Design review of the part built by this model. Coordinates are the model's own, in mm. A direction names the side the tool comes from. Coordinates: 2 decimals unless noted, no trailing zeros. Write each loop counter-clockwise with the first axis right and the second up, starting at its lowest first coordinate (ties: lowest second). Pieces come first, ordered by that corner, then holes. Notation, with made-up numbers: (-37.75, 23) - (4.25, 23) arc R22 cw to (4.25, 57) - close; hole circle Ø6 at (45, 54.25). An arc over 180 degrees is marked (long way). Answer as CSV lines item,"result". Start each with the question number.
Q1. Mouldability with a two-part tool opening along Y and no side actions: class faces 4 (the face through (25, -15, 5)), 5 (the face through (-15, -25, 5)), 6 (the face through (-19, -8, 5)) as pulls with the +Y half, pulls with the -Y half, needs draft (parallel to the pull), parting line crosses it, or undercut.
Q2. For line 1 along X through (y, z) = (-18.5, 5); line 2 along Y through (x, z) = (8, 7.25), list the stretches that pass through material, from the lowest coordinate up. Write a range as [from, to].
Q3. Machinability: for faces 1 (the face through (-5.1, -22, 5)), 2 (the face through (15, -25, 5)), 3 (the face through (-10.5, -17, 5)), which of the approach directions +Z, -Z, +X, -X, +Y, -Y give a long, thin tool a straight path to every point of the face, cutting with its end or side? Answer none if there is none.
Q4. We need section A-A (y = 20.5). Write out the cut boundary in (x, z), plus the area to 3 significant figures.
Q5. Clearance check with a flat-ended pin moving along its axis: pin 1 (6 mm diameter, centred on x = 0, z = 2.5, fed in from +Y). State where the tip first meets the part, or that it passes through.
Q6. We need section B-B (x = -18). Write out the cut boundary in (y, z).
Autodesk Inventor part; units mm, degrees
ref_plane "YZ Plane" through (0, 0, 0) normal (1, 0, 0) x (0, 1, 0)
ref_plane "XZ Plane" through (0, 0, 0) normal (0, 1, 0) x (-1, 0, 0)
ref_plane "XY Plane" through (0, 0, 0) normal (0, 0, 1) x (1, 0, 0)
sketch "Sketch2" plane through (0, 0, 0) normal (0, 0, 1) x (1, 0, 0)
  line L0 (0, 0) -> (0, 6) construction
  circle A0 centre (0, 0) radius 6 construction
  circle A1 centre (0, 0) radius 7 construction
  arc A2 (1.1705, 5.8847) -> (-1.1705, 5.8847) centre (0, 0) ccw
  line L1 (-1.3656, 6.8655) -> (0, 0) construction
  line L2 (-1.3656, 6.8655) -> (-1.1705, 5.8847)
  arc A3 (-1.3656, 6.8655) -> (-3.889, 5.8203) centre (0, 0) ccw
  line L3 (0, 0) -> (-3.889, 5.8203) construction
  line L4 (-3.889, 5.8203) -> (-3.3334, 4.9888)
  line L5 (-6.8655, 1.3656) -> (-5.8847, 1.1705)
  arc A4 (-5.8203, 3.889) -> (-6.8655, 1.3656) centre (0, 0) ccw
  line L6 (-5.8203, 3.889) -> (-4.9888, 3.3334)
  arc A5 (-3.3334, 4.9888) -> (-4.9888, 3.3334) centre (0, 0) ccw
  line L7 (-5.8203, -3.889) -> (-4.9888, -3.3334)
  arc A6 (-6.8655, -1.3656) -> (-5.8203, -3.889) centre (0, 0) ccw
  line L8 (-6.8655, -1.3656) -> (-5.8847, -1.1705)
  arc A7 (-5.8847, 1.1705) -> (-5.8847, -1.1705) centre (0, 0) ccw
  line L9 (-1.3656, -6.8655) -> (-1.1705, -5.8847)
  arc A8 (-3.889, -5.8203) -> (-1.3656, -6.8655) centre (0, 0) ccw
  line L10 (-3.889, -5.8203) -> (-3.3334, -4.9888)
  arc A9 (-4.9888, -3.3334) -> (-3.3334, -4.9888) centre (0, 0) ccw
  line L11 (3.889, -5.8203) -> (3.3334, -4.9888)
  arc A10 (1.3656, -6.8655) -> (3.889, -5.8203) centre (0, 0) ccw
  line L12 (1.3656, -6.8655) -> (1.1705, -5.8847)
  arc A11 (-1.1705, -5.8847) -> (1.1705, -5.8847) centre (0, 0) ccw
  line L13 (6.8655, -1.3656) -> (5.8847, -1.1705)
  arc A12 (5.8203, -3.889) -> (6.8655, -1.3656) centre (0, 0) ccw
  line L14 (5.8203, -3.889) -> (4.9888, -3.3334)
  arc A13 (3.3334, -4.9888) -> (4.9888, -3.3334) centre (0, 0) ccw
  line L15 (5.8203, 3.889) -> (4.9888, 3.3334)
  arc A14 (6.8655, 1.3656) -> (5.8203, 3.889) centre (0, 0) ccw
  line L16 (6.8655, 1.3656) -> (5.8847, 1.1705)
  arc A15 (5.8847, -1.1705) -> (5.8847, 1.1705) centre (0, 0) ccw
  line L17 (1.3656, 6.8655) -> (1.1705, 5.8847)
  arc A16 (3.889, 5.8203) -> (1.3656, 6.8655) centre (0, 0) ccw
  line L18 (3.889, 5.8203) -> (3.3334, 4.9888)
  arc A17 (4.9888, 3.3334) -> (3.3334, 4.9888) centre (0, 0) ccw
  circle A18 centre (0, 0) radius 12
  line L19 (-20.9, 20.9) -> (-14.1, 20.9) construction
  line L20 (-14.1, 20.9) -> (-14.1, 14.1) construction
  line L21 (-14.1, 14.1) -> (-20.9, 14.1) construction
  line L22 (-20.9, 14.1) -> (-20.9, 20.9) construction
  line L23 (-20.9, 20.9) -> (-14.1, 14.1) construction
  line L24 (-14.1, 20.9) -> (-20.9, 14.1) construction
  line L25 (-21.5, 13.5) -> (-13.5, 13.5) construction
  line L26 (-13.5, 13.5) -> (-13.5, 21.5) construction
  line L27 (-13.5, 21.5) -> (-21.5, 21.5) construction
  line L28 (-21.5, 21.5) -> (-21.5, 13.5) construction
  line L29 (-21.5, 13.5) -> (-13.5, 21.5) construction
  line L30 (-13.5, 13.5) -> (-21.5, 21.5) construction
  line L31 (-19, 20.9) -> (-16, 20.9)
  line L32 (-19, 20.9) -> (-19, 21.5)
  line L33 (-25, 25) -> (-25, 5.1)
  line L34 (-25, 25) -> (-5.1, 25)
  line L35 (-25, 5.1) -> (-19, 5.1)
  line L36 (-19, 5.1) -> (-19, 10.5)
  line L37 (-19, 10.5) -> (-12, 10.5) construction
  line L38 (-12, 0) -> (-12, 10.5) construction
  arc A19 (-11.2123, 4.276) -> (-15.5, 10.5) centre (-15.5, 5.9111) ccw
  line L39 (-19, 10.5) -> (-15.5, 10.5)
  line L40 (-5.1, 25) -> (-5.1, 19)
  line L41 (-5.1, 19) -> (-10.5, 19)
  line L42 (-10.5, 19) -> (-10.5, 15.5)
  arc A20 (-10.5, 15.5) -> (-4.276, 11.2123) centre (-5.9111, 15.5) ccw
  point P0 (-4.2426, 4.2426)
  point P1 (-6, 0)
  point P2 (-4.2426, -4.2426)
  point P3 (0, -6)
  point P4 (4.2426, -4.2426)
  point P5 (6, 0)
  point P6 (4.2426, 4.2426)
  point P7 (-5.8847, 1.1705)
  point P8 (-3.3334, 4.9888)
  point P9 (1.1705, 5.8847)
  point P10 (4.9888, 3.3334)
  point P11 (-1.1705, -5.8847)
  point P12 (-4.9888, -3.3334)
  point P13 (-17.5, 17.5)
  point P14 (-17.5, 20.9)
  dimension "d1" = 14
  dimension "d2" = 12
  dimension "d7" = 360
  dimension "d10" = 22.5
  dimension "d11" = 24
  dimension "d14" = 17.5
  dimension "d15" = 17.5
  dimension "d16" = 6.8
  dimension "d17" = 8
  dimension "d18" = 3
  dimension "d19" = 25
  dimension "d20" = 5.1
  dimension "d21" = 25
  dimension "d22" = 6
  dimension "d23" = 3
extrude "Extrusion1" add sketch "Sketch2" along normal blind 10 contours A18
extrude "Extrusion2" add sketch "Sketch2" along normal blind 10 contours A18 A19 L39 L36 L35 L33 L34 L40 L41 L42 A20
pattern_circular "Circular Pattern2" count 4 over 360 about axis through (0, 0, 0) along (0, 0, 1) of "Extrusion2"
properties part number "Perfil-de-aluminio-0001-002" material "Aluminum 6061"
Results list:
1,face 4,"needs draft"
1,face 5,"pulls with the -Y half"
1,face 6,"undercut"
2,line 1,"x = [-25, -10.5], [10.5, 25]"
2,line 2,"y = [-25, -19], [-11.41, 11.41], [19, 25]"
3,face 1,"+Z, -Z, -Y"
3,face 2,"+Z, -Z, +X, -X, -Y"
3,face 3,"+Z, -Z"
4,outline,"(-25, 0) - (-5.1, 0) - (-5.1, 10) - (-25, 10) - close; (5.1, 0) - (25, 0) - (25, 10) - (5.1, 10) - close"
4,area,"398 mm2"
5,pin 1,"stops at y = 12"
6,outline,"(-25, 0) - (-10.5, 0) - (-10.5, 10) - (-25, 10) - close; (10.5, 0) - (25, 0) - (25, 10) - (10.5, 10) - close"
